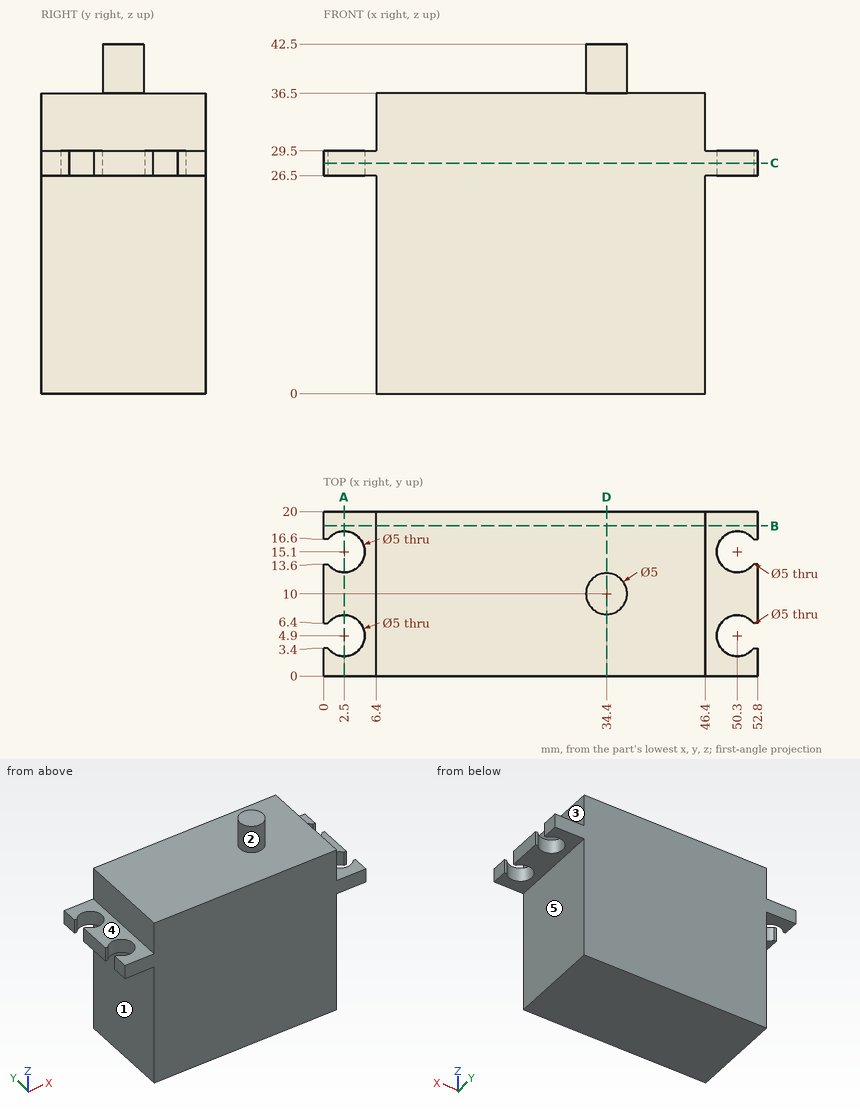
Input: dimensioned drawing with shaded views. Units: mm. Origin: part minimum x, y, z. A direction names the side the tool comes from. Round coordinates to 2 decimals unless told otherwise and drop trailing zeros. Loops run counter-clockwise (first coordinate to the right, second up) from the corner with the lowest first, then second, coordinate; pieces in that order, holes last. Notation, with made-up numbers: (54, 60.5) -> (92, 60.5) arc R29 ccw to (92, 97.5) -> close; hole circle Ø2 at (18, 58). An arc over 180 degrees is marked (long way). Answer as a JSON object with one key per item and string values. Group by question number.
Q1. Section query C-C (z = 28). Output: boundary loops of the cut face in (x, y).
Q2. Section query D-D (x = 34.4). Output: boundary loops of the cut face in (y, z), plus the area to 3 significant figures.
Q3. Contact query for flat-ended pins moving along their axis: P1, Ø8, axis at x = 50.3, y = 15.1, coming from the +Z side; P2, Ø5, axis at x = 49, y = 10, coming from the -Z side; P3, Ø1, axis at y = 10, z = 30.5, coming from the -X side; P4, Ø12, axis at x = 21, y = 16, coming from the -Z side. Output: stop coordinate, or through.
Q4. Ray query, line 1 (Y direction, x = 50.3, z = 27.5); line 2 (Y direction, x = 2, z = 28); line 3 (X direction, y = 18.25, z = 22.5). Return the intervals inside material, ascending. Write a range as from..to.
Q5. Section query B-B (y = 18.25). Output: boundary loops of the cut face in (x, z).
Q6. Section query A-A (x = 2.5). Output: boundary loops of the cut face in (y, z).
Q7. Access query for the marked faces 1, 2, 3, 4 and 5. Directions: +Z, -Z, +X, -X, +Y, -Y. A direction counts if a zero-diameter tool reaches every point of the face in a straight line with its end or side. Return the directions, or none.
Completed:
{
 "1": {"outline": "(0, 0) -> (52.8, 0) -> (52.8, 3.4) -> (52.3, 3.4) arc R2.5 cw (long way) to (52.3, 6.4) -> (52.8, 6.4) -> (52.8, 13.6) -> (52.3, 13.6) arc R2.5 cw (long way) to (52.3, 16.6) -> (52.8, 16.6) -> (52.8, 20) -> (0, 20) -> (0, 16.6) -> (0.5, 16.6) arc R2.5 cw (long way) to (0.5, 13.6) -> (0, 13.6) -> (0, 6.4) -> (0.5, 6.4) arc R2.5 cw (long way) to (0.5, 3.4) -> (0, 3.4) -> close"},
 "2": {"outline": "(0, 0) -> (20, 0) -> (20, 36.5) -> (12.5, 36.5) -> (12.5, 42.5) -> (7.5, 42.5) -> (7.5, 36.5) -> (0, 36.5) -> close", "area": "760 mm²"},
 "3": {"P1": "z = 36.5", "P2": "z = 26.5", "P3": "x = 6.4", "P4": "z = 0"},
 "4": {"line 1": "0..2.4, 7.4..12.6, 17.6..20", "line 2": "0..2.45, 7.35..12.65, 17.55..20", "line 3": "6.4..46.4"},
 "5": {"outline": "(0, 26.5) -> (6.4, 26.5) -> (6.4, 0) -> (46.4, 0) -> (46.4, 26.5) -> (52.8, 26.5) -> (52.8, 29.5) -> (46.4, 29.5) -> (46.4, 36.5) -> (6.4, 36.5) -> (6.4, 29.5) -> (0, 29.5) -> close"},
 "6": {"outline": "(0, 26.5) -> (2.4, 26.5) -> (2.4, 29.5) -> (0, 29.5) -> close; (7.4, 26.5) -> (12.6, 26.5) -> (12.6, 29.5) -> (7.4, 29.5) -> close; (17.6, 26.5) -> (20, 26.5) -> (20, 29.5) -> (17.6, 29.5) -> close"},
 "7": {"face 1": "-Z, -X, +Y, -Y", "face 2": "+Z", "face 3": "+Z, +X, +Y, -Y", "face 4": "+Z, -X, +Y, -Y", "face 5": "-Z, +X, +Y, -Y"}
}
